Check sheet for the modelled part. Datum: model origin and axes. Units: mm. Face numbers are marked on the shaded views. A direction names the side the tool comes from. Give positions to 0.01 mm unless a question says otherwise; leave off trailing zeros. Order: outer loops, then holes, each group sorted by start corner. A loop starts at its lowest first (then second) coordinate and runs counter-clockwise, first axis right, second up. Notation, with made-up numbers: (-13, 24) - (9, 24) arc R28 ccw to (9, 42) - close; hole circle Ø4 at (-15, -19.5). An arc over 180 degrees is marked (long way). Answer in a Markdown table with one row per item.
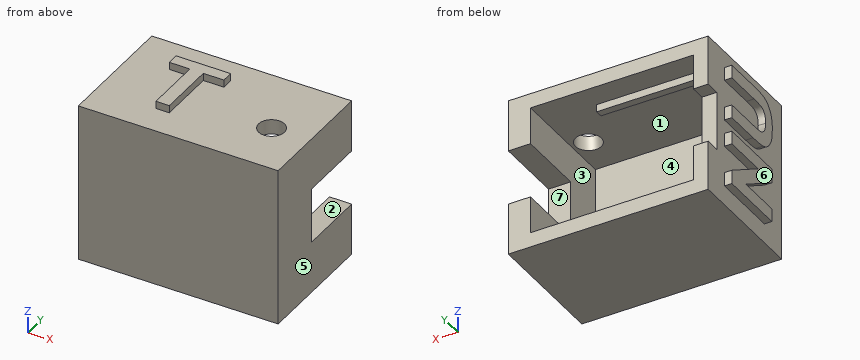
from build123d import *

# Parameters (mm, degrees)
SKETCH1_W           = 27
SKETCH1_H           = 21.5
BOSS_EXTRUDE1_DEPTH = 2
SKETCH2_W           = 27
SKETCH2_H           = 21.5
SKETCH2_W_2         = 22
SKETCH2_H_2         = 17.5
BOSS_EXTRUDE2_DEPTH = 15
SKETCH3_W           = 15
SKETCH3_H           = 1.5
BOSS_EXTRUDE3_DEPTH = 1
SKETCH4_W           = 15
SKETCH4_H           = 1
BOSS_EXTRUDE4_DEPTH = 1
SKETCH7_R           = 1.75
CUT_EXTRUDE2_DEPTH  = 2
SKETCH8_W           = 3
SKETCH8_H           = 7.46
CUT_EXTRUDE3_DEPTH  = 9.3
BOSS_EXTRUDE5_DEPTH = 1
BOSS_EXTRUDE6_DEPTH = 1
SKETCH11_W          = 2
SKETCH11_H          = 8
CUT_EXTRUDE4_DEPTH  = 2


with BuildPart() as part:
    # Sketch1 → Boss-Extrude1 (new body)
    with BuildSketch(Plane(origin=(0, 0, 0), x_dir=(1, 0, 0), z_dir=(0, 1, 0))):
        with Locations((7.695979899, -3.494974874)):
            Rectangle(SKETCH1_W, SKETCH1_H)
    extrude(amount=BOSS_EXTRUDE1_DEPTH)

    # Sketch2 → Boss-Extrude2 (add)
    with BuildSketch(Plane(origin=(0, 2, 0), x_dir=(1, 0, 0), z_dir=(0, 1, 0))):
        with Locations((7.695979899, -3.494974874)):
            Rectangle(SKETCH2_W, SKETCH2_H)
        with Locations((7.195979899, -3.494974874)):
            Rectangle(SKETCH2_W_2, SKETCH2_H_2, mode=Mode.SUBTRACT)
    extrude(amount=BOSS_EXTRUDE2_DEPTH)

    # Sketch3 → Boss-Extrude3 (add)
    with BuildSketch(Plane.XY.offset(-5.255025126)):
        with Locations((3.695979899, 12.95)):
            Rectangle(SKETCH3_W, SKETCH3_H)
    extrude(amount=BOSS_EXTRUDE3_DEPTH)

    # Sketch4 → Boss-Extrude4 (add)
    with BuildSketch(Plane(origin=(0, 0, 12.244974874), x_dir=(-1, 0, 0), z_dir=(0, 0, -1))):
        with Locations((-3.695979899, 13.2)):
            Rectangle(SKETCH4_W, SKETCH4_H)
    extrude(amount=BOSS_EXTRUDE4_DEPTH)

    # Sketch7 → Cut-Extrude2 (cut)
    with BuildSketch(Plane.XY.offset(14.244974874)):
        with Locations((16.00290807, 7.361856015)):
            Circle(SKETCH7_R)
    extrude(amount=-CUT_EXTRUDE2_DEPTH, mode=Mode.SUBTRACT)

    # Sketch8 → Cut-Extrude3 (cut)
    with BuildSketch(Plane(origin=(0, 17, 0), x_dir=(1, 0, 0), z_dir=(0, 1, 0))):
        with Locations((19.695979899, -3.494974874)):
            Rectangle(SKETCH8_W, SKETCH8_H)
    extrude(amount=-CUT_EXTRUDE3_DEPTH, mode=Mode.SUBTRACT)

    # Sketch9 → Boss-Extrude5 (add)
    with BuildSketch(Plane.ZY.offset(5.804020101)):
        Polygon((-4.61402787, 3.994511949), (-4.61402787, 13.240459214), (-2.756318514, 13.240459214), (0.957248046, 7.16539771), (0.957248046, 13.240459214), (2.735314828, 13.240459214), (2.735314828, 3.994511949), (0.822040884, 3.994511949), (-2.835961089, 9.976965808), (-2.835961089, 3.994511949), align=None)
        with BuildLine():
            Line((4.631919395, 13.240459214), (6.409986177, 13.240459214))
            Line((6.409986177, 13.240459214), (6.409986177, 8.222977014))
            add(Edge.make_bspline(
                [(6.409986177, 8.222977014), (6.410664977, 8.127899938), (6.411960871, 7.946388772), (6.412852908, 7.687065219), (6.417789545, 7.454232779), (6.428495129, 7.247516275), (6.435842667, 7.067021131), (6.449486246, 6.912714219), (6.46309676, 6.784655632), (6.476329448, 6.708485325), (6.48222014, 6.674577192)],
                knots=[0, 0, 0, 0, 0.000285238, 0.000544546, 0.000777983, 0.00098378, 0.001165528, 0.001319802, 0.001448457, 0.00155168, 0.00155168, 0.00155168, 0.00155168], degree=3))
            add(Edge.make_bspline(
                [(6.48222014, 6.674577192), (6.506506, 6.583165819), (6.554327924, 6.403165284), (6.686142733, 6.157109332), (6.860268235, 5.940226506), (7.037882666, 5.785554138), (7.198548601, 5.676088514), (7.335021148, 5.609466156), (7.47981763, 5.548735594), (7.63599912, 5.502137547), (7.801889384, 5.46136258), (7.979492203, 5.437786208), (8.167308711, 5.419691929), (8.296044968, 5.417890479), (8.362155331, 5.416965374)],
                knots=[0, 0, 0, 0, 0.000282968, 0.000557199, 0.000829969, 0.001113451, 0.001260368, 0.00141195, 0.001568103, 0.001730967, 0.001900335, 0.002080022, 0.002267831, 0.002466089, 0.002466089, 0.002466089, 0.002466089], degree=3))
            add(Edge.make_bspline(
                [(8.362155331, 5.416965374), (8.42885346, 5.41817507), (8.558713354, 5.420530322), (8.74690251, 5.434556672), (8.922479775, 5.46101956), (9.085337742, 5.495717516), (9.23633657, 5.539569917), (9.374271612, 5.595092211), (9.498925505, 5.661908259), (9.645391949, 5.762616554), (9.802989652, 5.904683185), (9.954657319, 6.097840917), (10.063204683, 6.311066042), (10.114117997, 6.505756529), (10.140285731, 6.675384373), (10.156228521, 6.823814626), (10.170809009, 6.99178617), (10.184049207, 7.178838934), (10.193103805, 7.385113322), (10.198001278, 7.611131016), (10.201855616, 7.856855971), (10.202738101, 8.027264527), (10.203195312, 8.115552146)],
                knots=[0, 0, 0, 0, 0.00020011, 0.000389609, 0.000565632, 0.000732377, 0.000888849, 0.001036743, 0.001177616, 0.001312213, 0.001569242, 0.001810797, 0.00204521, 0.002281568, 0.00241098, 0.002560087, 0.002729283, 0.0029168, 0.003122597, 0.003348628, 0.003594992, 0.003859856, 0.003859856, 0.003859856, 0.003859856], degree=3))
            Line((10.203195312, 8.115552146), (10.203195312, 13.240459214))
            Line((10.203195312, 13.240459214), (11.981262093, 13.240459214))
            Line((11.981262093, 13.240459214), (11.981262093, 8.404487998))
            add(Edge.make_bspline(
                [(11.981262093, 8.404487998), (11.981034195, 8.271131655), (11.980596294, 8.014891106), (11.973759084, 7.646224887), (11.959227844, 7.307989087), (11.947059184, 6.999603918), (11.923586339, 6.721856103), (11.89901035, 6.47457295), (11.867350881, 6.257797674), (11.822204183, 6.011401071), (11.746332221, 5.734959937), (11.624052705, 5.42959525), (11.467775809, 5.151778752), (11.278124263, 4.900444487), (11.056190615, 4.674593522), (10.798651876, 4.475113752), (10.508156306, 4.299580065), (10.241950666, 4.173184842), (10.009853453, 4.08807444), (9.820814155, 4.030475534), (9.61849876, 3.982507696), (9.403144549, 3.94444095), (9.174658985, 3.912345052), (8.932959111, 3.890910251), (8.678410596, 3.877533423), (8.50478883, 3.876502272), (8.415867765, 3.875974163)],
                knots=[0, 0, 0, 0, 0.000400069, 0.000768722, 0.001106063, 0.001415727, 0.001694438, 0.001942135, 0.002161113, 0.002351461, 0.002693408, 0.003019119, 0.003335923, 0.003646716, 0.003961047, 0.004283013, 0.004621309, 0.004977577, 0.005165094, 0.005362546, 0.005570094, 0.005788436, 0.006018417, 0.006262065, 0.00651614, 0.006782876, 0.006782876, 0.006782876, 0.006782876], degree=3))
            add(Edge.make_bspline(
                [(8.415867765, 3.875974163), (8.309052797, 3.877339536), (8.10213628, 3.879984467), (7.801779753, 3.891783276), (7.521923904, 3.916136469), (7.261689478, 3.94905209), (7.02118392, 3.991366197), (6.799798809, 4.041952447), (6.59930158, 4.105886329), (6.360493291, 4.19719937), (6.094301616, 4.336877712), (5.804540716, 4.523207483), (5.550180475, 4.733513713), (5.333455831, 4.965741446), (5.152282464, 5.211729672), (5.005020527, 5.466155478), (4.887009657, 5.724778163), (4.837698017, 5.904525991), (4.813430379, 5.992984925)],
                knots=[0, 0, 0, 0, 0.000320471, 0.000620799, 0.000901509, 0.001162945, 0.001407464, 0.001633889, 0.0018436, 0.002038279, 0.002400265, 0.002742918, 0.003070414, 0.003387527, 0.003693514, 0.003984821, 0.004268412, 0.004543212, 0.004543212, 0.004543212, 0.004543212], degree=3))
            add(Edge.make_bspline(
                [(4.813430379, 5.992984925), (4.79857773, 6.062627668), (4.767293301, 6.209317553), (4.731762874, 6.442525714), (4.699348655, 6.699326958), (4.677209321, 6.980025037), (4.65622326, 7.283729346), (4.64115601, 7.611012524), (4.634960344, 7.961800253), (4.632953465, 8.203837094), (4.631919395, 8.328549729)],
                knots=[0, 0, 0, 0, 0.000213585, 0.000449878, 0.000707407, 0.000989962, 0.001294397, 0.001620713, 0.0019727, 0.002346853, 0.002346853, 0.002346853, 0.002346853], degree=3))
            Line((4.631919395, 8.328549729), (4.631919395, 13.240459214))
        make_face()
    extrude(amount=BOSS_EXTRUDE5_DEPTH)

    # Sketch10 → Boss-Extrude6 (add)
    with BuildSketch(Plane.XY.offset(14.244974874)):
        Polygon((2.278412827, 4.103597224), (2.278412827, 11.963582575), (-0.502812759, 11.963582575), (-0.502812759, 13.535579645), (6.873481186, 13.535579645), (6.873481186, 11.963582575), (4.0922556, 11.963582575), (4.0922556, 4.103597224), align=None)
    extrude(amount=BOSS_EXTRUDE6_DEPTH)

    # Sketch11 → Cut-Extrude4 (cut)
    with BuildSketch(Plane(origin=(0, 17, 0), x_dir=(1, 0, 0), z_dir=(0, 1, 0))):
        with Locations((-4.804020101, -3.494974874)):
            Rectangle(SKETCH11_W, SKETCH11_H)
    extrude(amount=-CUT_EXTRUDE4_DEPTH, mode=Mode.SUBTRACT)


solid = part.part
(1) Gauge pin test, flat ends, axial feed: P1, Ø1.1, axis at x = -6.5, y = 8.5, coming from the +Z side; P2, Ø1, axis at x = 9, z = 1, coming from the +Y side; P3, Ø0.8, axis at x = 5, z = 15, coming from the -Y side; P4, Ø12, axis at x = 14.5, z = 1.5, coming from the -Y side. Record the tip position at first contact, or that the pin passes through.
Geometry says:
| item | result |
|---|---|
| P1 | z = 11.98 |
| P2 | y = 2 |
| P3 | y = 11.96 |
| P4 | y = 0 |
(2) Cross-section at B-B, the plane x = 16.75. Record the cut outline in (y, z), then the cut area to 3 significant figures.
Geometry says:
| item | result |
|---|---|
| outline | (0, -7.26) - (17, -7.26) - (17, -5.26) - (2, -5.26) - (2, 12.24) - (5.78, 12.24) - (5.78, 14.24) - (0, 14.24) - close; (8.94, 12.24) - (17, 12.24) - (17, 14.24) - (8.94, 14.24) - close |
| area | 96.7 mm² |
(3) Cross-section at A-A, the plane x = 0.75. Record the cut outline in (y, z).
Geometry says:
| item | result |
|---|---|
| outline | (0, -7.26) - (17, -7.26) - (17, -5.26) - (13.7, -5.26) - (13.7, -4.26) - (12.2, -4.26) - (12.2, -5.26) - (2, -5.26) - (2, 12.24) - (12.7, 12.24) - (12.7, 11.24) - (13.7, 11.24) - (13.7, 12.24) - (17, 12.24) - (17, 14.24) - (13.54, 14.24) - (13.54, 15.24) - (11.96, 15.24) - (11.96, 14.24) - (0, 14.24) - close |
(4) Cross-section at D-D, the plane x = 12.75. Record the cut outline in (y, z), then the cut area to 3 significant figures.
Geometry says:
| item | result |
|---|---|
| outline | (0, -7.26) - (17, -7.26) - (17, -5.26) - (2, -5.26) - (2, 12.24) - (17, 12.24) - (17, 14.24) - (0, 14.24) - close |
| area | 103 mm² |
(5) Thickness scan on L1, parallel to X at y = 5, z = 10; L2, parallel to X at y = 3.75, z = 10.25; L3, parallel to Z at x = 17.5, y = 5. Record the ranges inside material, lowest first.
Geometry says:
| item | result |
|---|---|
| L1 | -6.8 to -3.8, 18.2 to 21.2 |
| L2 | -5.8 to -3.8, 18.2 to 21.2 |
| L3 | -7.26 to -5.26, 12.24 to 14.24 |
(6) Mould release check, pull along X, two halves, no side actions. Record for the marked faces 4, 5, 6 and 7: pulls with the +X half, pulls with the -X half, needs draft (parallel to the pull), parting line crosses it, or undercut.
Geometry says:
| item | result |
|---|---|
| face 4 | undercut |
| face 5 | pulls with the +X half |
| face 6 | pulls with the -X half |
| face 7 | needs draft |
(7) Access from +Z, -Z, +X, -X, +Y, -Y to the whole of each face (thin tool, end or side, straight path). Record for the marked faces 1, 2 and 3.
Geometry says:
| item | result |
|---|---|
| face 1 | none |
| face 2 | +X, +Y |
| face 3 | +Y |
